Can you work these out from the model? Positions are in its coordinate system, mm. Face numbers are marked on the shaded views. A direction names the side the tool comes from. Round coordinates to 2 decimals unless told otherwise and drop trailing zeros. Loops run counter-clockwise (first coordinate to the right, second up) from the corner with the lowest first, then second, coordinate; pieces in that order, holes last. Notation, with made-up numbers: M -33,79.25 L 7,79.25 A28 cw 7,98.25 Z; hole C 4,51.5 d9. An arc over 180 degrees is marked long. Return JSON: item names as keys, results as strings.
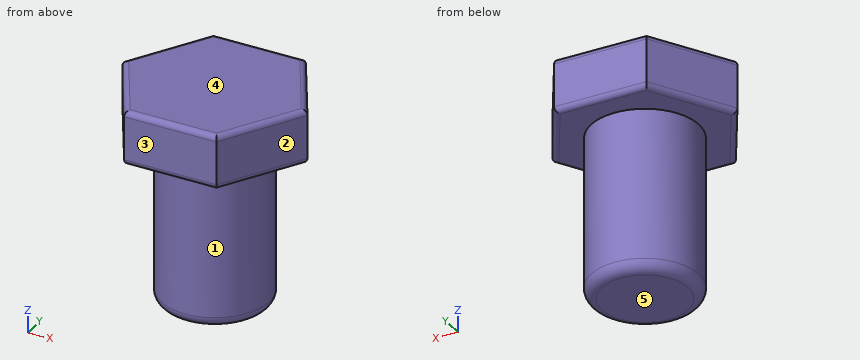
```python
from build123d import *

# Parameters (mm, degrees)
SKETCH_1_R      = 5
EXTRUDE_1_DEPTH = 15
EXTRUDE_2_DEPTH = 5
FILLET_1_R      = 0.5
FILLET_2_R      = 1


with BuildPart() as part:
    # 草图1 → 凸台-拉伸1 (new body)
    with BuildSketch(Plane.XY):
        Circle(SKETCH_1_R)
    extrude(amount=EXTRUDE_1_DEPTH)

    # 草图2 → 凸台-拉伸2 (add)
    with BuildSketch(Plane.XY.offset(15)):
        Polygon((4.330127019, -7.5), (8.660254038, 0), (4.330127019, 7.5), (-4.330127019, 7.5), (-8.660254038, 0), (-4.330127019, -7.5), align=None)
    extrude(amount=EXTRUDE_2_DEPTH)

    # 圆角1
    fillet_1_edges = [part.edges().sort_by_distance(p)[0] for p in [
        (0, -7.5, 15),
        (6.495190528, -3.75, 15),
        (6.495190528, 3.75, 15),
        (0, 7.5, 15),
        (-6.495190528, 3.75, 15),
        (-6.495190528, -3.75, 15),
        (0, -7.5, 20),
        (6.495190528, -3.75, 20),
        (6.495190528, 3.75, 20),
        (0, 7.5, 20),
        (-6.495190528, 3.75, 20),
        (-6.495190528, -3.75, 20),
    ]]
    fillet(fillet_1_edges, radius=FILLET_1_R)

    # 圆角2
    fillet_2_edges = [part.edges().sort_by_distance(p)[0] for p in [
        (-5, 0, 0),
    ]]
    fillet(fillet_2_edges, radius=FILLET_2_R)


solid = part.part
```
Q1. Suppose I cut it at A-A, the plane x = 0. Please give me the cut outline in (y, z).
Results:
{"outline": "M -7.5,15.5 A0.5 ccw -7,15 L -5,15 L -5,1 A1 ccw -4,0 L 4,0 A1 ccw 5,1 L 5,15 L 7,15 A0.5 ccw 7.5,15.5 L 7.5,19.5 A0.5 ccw 7,20 L -7,20 A0.5 ccw -7.5,19.5 Z"}
Q2. On a 3-axis mill with a long thin cutter (end or side, diameter ignored), from which of +Z, -Z, +X, -X, +Y, -Y can I reach the whole of each face in a straight line? I mean the marked faces 1 and 2. Say none if no direction works.
Results:
{"face 1": "-Z", "face 2": "+Z, -Z, +X, -Y"}
Q3. If I drill on line 1 along X through (y, z) = (1, 15.5); line 2 along Z through (x, y) = (-6.25, -2.75); line 3 along X through (y, z) = (3, 8.75), over which ranges is the centre line in solid material (lowest first)?
Results:
{"line 1": "x = -8.08 to 8.08", "line 2": "z = 15 to 20", "line 3": "x = -4 to 4"}
Q4. Thinking about a two-plate mould opening in Z: for the marked faces 3, 4 and 5, which applies, pulls with the +Z half, pulls with the -Z half, needs draft (parallel to the pull), parting line crosses it, or undercut?
Results:
{"face 3": "needs draft", "face 4": "pulls with the +Z half", "face 5": "pulls with the -Z half"}
Q5. Suppose I cut it at B-B, the plane z = 6.75. Please give me the cut outline in (x, y).
Results:
{"outline": "C 0,0 d10"}
Q6. I'm going to push flat-ended pins straight in: pin 1 Ø2 at (y, z) = (3, 3) entering from -X; pin 2 Ø6 at (x, z) = (-3, 6.5) entering from -Y; pin 3 Ø5 at (y, z) = (5.5, 18) entering from -X. Where does each tip first touch, or does it pass through?
Results:
{"pin 1": "stops at x = -4.58", "pin 2": "stops at y = -5", "pin 3": "stops at x = -6.93"}
